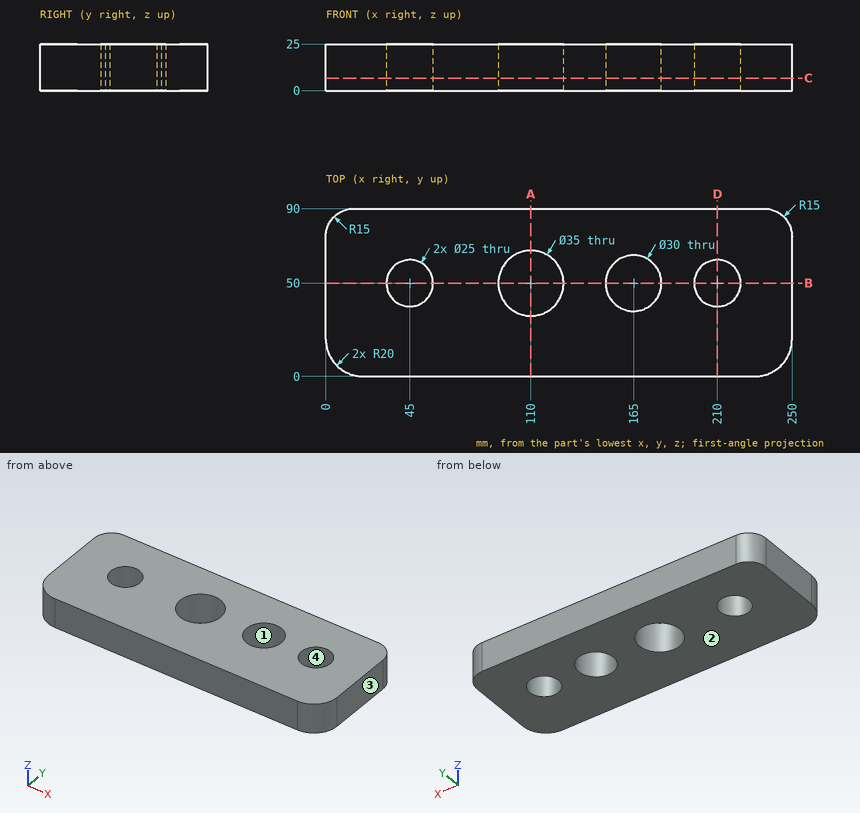
Here's the drawing with two shaded views (mm, measured from the low corner). I have some questions. Give positions to 0.01 mm unless a question says otherwise; leave off trailing zeros. Order: outer loops, then holes, each group sorted by start corner. A loop starts at its lowest first (then second) coordinate and runs counter-clockwise, first axis right, second up. Notation, with made-up numbers: M 54,-4 L 92,-4 A15 ccw 92,0 Z; hole C 61.5,67 d7. An arc over 180 degrees is marked long. Answer as a JSON object with one key per item and string values. Group by question number.
1) Suppose I cut it at B-B, the plane y = 50. Write out the boundary of the cut face in (x, z).
2) We'd pull the mould along X, two halves only. Please class the marked faces 1, 2, 3 and 4: pulls with the +X half, pulls with the -X half, needs draft (parallel to the pull), parting line crosses it, or undercut.
3) Please list where these lines run through material, in increasing order: L1, parallel to Y at x = 210, z = 5; L2, parallel to Y at x = 110, z = 18.5; L3, parallel to X at y = 55.5, z = 4.25. Write a range as [from, to].
4) Suppose I cut it at D-D, the plane x = 210. Write out the boundary of the cut face in (y, z).
5) Suppose I cut it at A-A, the plane x = 110. Write out the boundary of the cut face in (y, z), plus the area to 4 significant figures.
6) Suppose I cut it at C-C, the plane z = 6.75. Write out the boundary of the cut face in (x, y).
Results found:
{
 "1": {"outline": "M 0,0 L 32.5,0 L 32.5,25 L 0,25 Z; M 57.5,0 L 92.5,0 L 92.5,25 L 57.5,25 Z; M 127.5,0 L 150,0 L 150,25 L 127.5,25 Z; M 180,0 L 197.5,0 L 197.5,25 L 180,25 Z; M 222.5,0 L 250,0 L 250,25 L 222.5,25 Z"},
 "2": {"face 1": "undercut", "face 2": "needs draft", "face 3": "pulls with the +X half", "face 4": "undercut"},
 "3": {"L1": "[0, 37.5], [62.5, 90]", "L2": "[0, 32.5], [67.5, 90]", "L3": "[0, 33.78], [56.22, 93.39], [126.61, 151.04], [178.96, 198.78], [221.22, 250]"},
 "4": {"outline": "M 0,0 L 37.5,0 L 37.5,25 L 0,25 Z; M 62.5,0 L 90,0 L 90,25 L 62.5,25 Z"},
 "5": {"outline": "M 0,0 L 32.5,0 L 32.5,25 L 0,25 Z; M 67.5,0 L 90,0 L 90,25 L 67.5,25 Z", "area": "1,375 mm²"},
 "6": {"outline": "M 0,20 A20 ccw 20,0 L 230,0 A20 ccw 250,20 L 250,75 A15 ccw 235,90 L 15,90 A15 ccw 0,75 Z; hole C 45,50 d25; hole C 110,50 d35; hole C 165,50 d30; hole C 210,50 d25"}
}
